Check sheet for the modelled part. Datum: model origin and axes. Units: mm. A direction names the side the tool comes from. Coordinates: 2 decimals unless noted, no trailing zeros. Order: outer loops, then holes, each group sorted by start corner. A loop starts at its lowest first (then second) coordinate and runs counter-clockwise, first axis right, second up.
1. Thickness scan on line 1 (Y direction, x = -2, z = 0); line 2 (Y direction, x = -6.5, z = 1.75); line 3 (Z direction, x = 2, y = -38). Record the ranges inside material, lowest first.
2. Gauge pin test, flat ends, axial feed: pin 1 Ø5 at (y, z) = (-32.5, -6) entering from +X; pin 2 Ø6 at (x, y) = (-3, -36) entering from -Z; pin 3 Ø10 at (x, z) = (-9.5, 2) entering from -Y; pin 4 Ø8 at (x, z) = (-6, -3) entering from -Y. Record the tip position at first contact, or that the pin passes through.
3. Cross-section at A-A (z = 0). Enter the section's corners in (x, y), then the cut area to 3 significant figures.
4. Cross-section at D-D (z = -7.5). Enter the section's corners in (x, y).
5. Set-up check for faces 1 (the flat face through (9, -0.424, 9)), 2 (the flat face through (0, 2.076, 0)), 3 (the flat face through (0, -3.924, 6)): record each of +Z, -Z, +X, -X, +Y, -Y from which the full face is reachable in a straight line by a thin tool's end or side.
6. Draft check along Y on faces 4 (the flat face through (0, -41.924, 0)), 5 (the flat face through (9, -1.424, -9)), 6 (the cylindrical face through (7.91, -2.692, -10.316)). Enter one of: released by +Y, released by -Y, zero draft, split by the parting line, or undercut.
7. Cross-section at C-C (x = 9.25). Enter the section's corners in (y, z).
8. Cross-section at B-B (x = 0). Enter the section's corners in (y, z), then the cut area to 3 significant figures.
```python
from build123d import *

# Parameters (mm, degrees)
SKETCH2_R                = 4.5
BOSS_EXTRUDE1_DEPTH      = 30
BOSS_EXTRUDE2_DEPTH      = 1
BOSS_EXTRUDE2_DEPTH_BACK = 1
CUT_EXTRUDE3_DEPTH       = 48.765956346
SKETCH6_R                = 4.5
BOSS_EXTRUDE3_DEPTH      = 8
CUT_EXTRUDE2_DEPTH       = 8
CUT_EXTRUDE2_DEPTH_BACK  = 47.071926172
SKETCH4_R                = 2.5
CUT_EXTRUDE5_START       = -8
SKETCH7_R                = 6.95034237
SKETCH7_R_2              = 4.5
CUT_EXTRUDE5_DEPTH       = 8


with BuildPart() as part:
    # Sketch1 → Revolve1 (revolve)
    with BuildSketch(Plane.XY, mode=Mode.PRIVATE) as revolve1_sk:
        Polygon((0, 2.075992783), (13, 2.075992783), (13, -0.424007217), (12, -0.424007217), (12, -1.424007217), (13, -1.424007217), (13, -3.924007217), (0, -3.924007217), align=None)
    revolve(revolve1_sk.sketch.rotate(Axis((0, 49.311920993, 0), (0, -1, 0)), 90), axis=Axis((0, 49.311920993, 0), (0, -1, 0)))

    # Sketch2 → Boss-Extrude1 (add)
    with BuildSketch(Plane.XZ.offset(3.924007217)):
        with Locations(Location((0, 0, 0), (0, 0, 270))):
            Circle(SKETCH2_R)
    extrude(amount=BOSS_EXTRUDE1_DEPTH)

    # Sketch3 → Boss-Extrude2 (add, two sides: drawn at the far end of the back side and taken through both)
    with BuildSketch(Plane(origin=(0, 0, 0), x_dir=(0, 0, -1), z_dir=(1, 0, 0)).offset(-BOSS_EXTRUDE2_DEPTH_BACK)):
        with BuildLine():
            Line((0, -33.924007217), (-4.5, -33.924007217))
            ThreePointArc((-4.5, -33.924007217), (-2.081257447, -43.403287407), (5.954829972, -37.824007217))
            ThreePointArc((5.954829972, -37.824007217), (5.57928019, -35.74274977), (4.5, -33.924007217))
            Line((4.5, -33.924007217), (0, -33.924007217))
        make_face()
    extrude(amount=BOSS_EXTRUDE2_DEPTH + BOSS_EXTRUDE2_DEPTH_BACK)

    # Sketch5 → Cut-Extrude3 (cut, through all)
    with BuildSketch(Plane(origin=(1, 0, 0), x_dir=(0, 0, -1), z_dir=(1, 0, 0))):
        with BuildLine():
            Line((5.205457264, -40.715929532), (-5.205457264, -40.715929532))
            ThreePointArc((-5.205457264, -40.715929532), (0, -43.77883719), (5.205457264, -40.715929532))
        make_face()
    extrude(amount=-CUT_EXTRUDE3_DEPTH, mode=Mode.SUBTRACT)

    # Sketch6 → Boss-Extrude3 (add)
    with BuildSketch(Plane.XZ.offset(33.924007217)):
        with Locations(Location((0, 0, 0), (0, 0, 270))):
            Circle(SKETCH6_R)
    extrude(amount=BOSS_EXTRUDE3_DEPTH)

    # Sketch4 → Cut-Extrude2 (cut, two sides: drawn at the far end of the back side and taken through both)
    with BuildSketch(Plane.ZY.offset(1).offset(-CUT_EXTRUDE2_DEPTH_BACK)):
        with Locations(Location((0, -37.824007217, 0), (0, 0, 180))):
            Circle(SKETCH4_R)
    extrude(amount=CUT_EXTRUDE2_DEPTH + CUT_EXTRUDE2_DEPTH_BACK, mode=Mode.SUBTRACT)

    # Sketch7 → Cut-Extrude5 (cut)
    with BuildSketch(Plane.XZ.offset(41.924007217).offset(CUT_EXTRUDE5_START)):
        Circle(SKETCH7_R)
        with Locations(Location((0, 0, 0), (0, 0, 270))):
            Circle(SKETCH7_R_2, mode=Mode.SUBTRACT)
    extrude(amount=CUT_EXTRUDE5_DEPTH, mode=Mode.SUBTRACT)


solid = part.part
```
Data:
1. line 1: y = -41.92 to -40.32, -35.32 to 2.08
1. line 2: y = -3.92 to 2.08
1. line 3: z = -4.03 to -2.49, 2.49 to 4.03
2. pin 1: stops at x = 2.83
2. pin 2: stops at z = -4.5
2. pin 3: stops at y = -3.92
2. pin 4: stops at y = -41.92
3. outline: (-13, -3.92) - (-4.5, -3.92) - (-4.5, -35.32) - (4.5, -35.32) - (4.5, -3.92) - (13, -3.92) - (13, -1.42) - (12, -1.42) - (12, -0.42) - (13, -0.42) - (13, 2.08) - (-13, 2.08) - (-13, -0.42) - (-12, -0.42) - (-12, -1.42) - (-13, -1.42) - close; (-4.5, -41.92) - (4.5, -41.92) - (4.5, -40.32) - (-4.5, -40.32) - close
3. area: 451 mm2
4. outline: (-10.62, -3.92) - (10.62, -3.92) - (10.62, -1.42) - (9.37, -1.42) - (9.37, -0.42) - (10.62, -0.42) - (10.62, 2.08) - (-10.62, 2.08) - (-10.62, -0.42) - (-9.37, -0.42) - (-9.37, -1.42) - (-10.62, -1.42) - close
5. face 1: none
5. face 2: +Z, -Z, +X, -X, +Y
5. face 3: -Y
6. face 4: released by -Y
6. face 5: undercut
6. face 6: zero draft
7. outline: (-3.92, -9.13) - (-1.42, -9.13) - (-1.42, -7.64) - (-0.42, -7.64) - (-0.42, -9.13) - (2.08, -9.13) - (2.08, 9.13) - (-0.42, 9.13) - (-0.42, 7.64) - (-1.42, 7.64) - (-1.42, 9.13) - (-3.92, 9.13) - close
8. outline: (-41.92, -4.5) - (-3.92, -4.5) - (-3.92, -13) - (-1.42, -13) - (-1.42, -12) - (-0.42, -12) - (-0.42, -13) - (2.08, -13) - (2.08, 13) - (-0.42, 13) - (-0.42, 12) - (-1.42, 12) - (-1.42, 13) - (-3.92, 13) - (-3.92, 4.5) - (-41.92, 4.5) - close; hole circle Ø5 at (-37.82, 0)
8. area: 476 mm2
